For this review, take the finished solid that the model builds, in its own axes (mm). A direction names the side the tool comes from. Round coordinates to 2 decimals unless told otherwise and drop trailing zeros. Loops run counter-clockwise (first coordinate to the right, second up) from the corner with the lowest first, then second, coordinate; pieces in that order, holes last. Notation, with made-up numbers: M -21.5,65.5 L -7.5,65.5 A27 ccw -7.5,94.5 Z; hole C 12.5,73 d6. An arc over 180 degrees is marked long. One line per question, with ' | ' between items. Start each with the question number.
1) For pin 1 Ø10 at (x, y) = (-11.5, -30) entering from +Z; pin 2 Ø1 at (x, z) = (-10, 48) entering from +Y; pin 3 Ø13.5 at (x, y) = (-6, 9.5) entering from +Z; pin 4 Ø10 at (x, y) = (-10.5, 26.5) entering from -Z, all flat-tipped, find the tip position at first contact; note any pin that passes through.
2) We need section D-D (x = -18). Give the boundary of the cut face in (y, z), and give its area (3 significant figures).
3) For probe 1 along Z at (x, y) = (-6.5, -12.5); probe 2 along Y at (x, z) = (5, 24); probe 3 along Y at (x, z) = (-5.5, 5.5), list the stretches that pass through material, from the lowest coordinate up. Write a range as from..to.
4) We need section C-C (x = 6.5). Give the boundary of the cut face in (y, z), and give its area (3 significant figures).
5) We need section A-A (z = 52). Give the boundary of the cut face in (x, y), and give its area (3 significant figures).
6) Mouldability with a two-part tool opening along Z and no side actions: class faces 3 (the face through (10, 0, 10)), 4 (the face through (0, -37.5, 43)), 5 (the face through (0, -9, 0)), 6 (the face through (-12.558, -41.198, 27.976)) as pulls with the +Z half, pulls with the -Z half, needs draft (parallel to the pull), parting line crosses it, or undercut.
7) We need section B-B (y = 7.5). Give the boundary of the cut face in (x, z), and give its area (3 significant figures).
8) For faces 1 (the face through (0, -41, 70)), 2 (the face through (12.558, -41.198, 27.976)), list the 3-axis set-ups (+Z, -Z, +X, -X, +Y, -Y) from which the entire face can be reached by the end or side of a thin tool; tool diameter is ignored.
```python
from build123d import *

# Parameters (mm, degrees)
SKETCH1_W           = 45
SKETCH1_H           = 90
BOSS_EXTRUDE1_DEPTH = 10
SKETCH2_R           = 16
CUT_EXTRUDE1_DEPTH  = 28
FILLET1_R           = 10
SKETCH3_W           = 45
SKETCH3_H           = 7.5
BOSS_EXTRUDE2_DEPTH = 60
FILLET2_R           = 7.5
CUT_EXTRUDE2_DEPTH  = 10


with BuildPart() as part:
    # Sketch1 → Boss-Extrude1 (new body)
    with BuildSketch(Plane.XY):
        Rectangle(SKETCH1_W, SKETCH1_H)
    extrude(amount=BOSS_EXTRUDE1_DEPTH)

    # Sketch2 → Cut-Extrude1 (cut)
    with BuildSketch(Plane.XY):
        with Locations((0.129474069, 13.005480981)):
            Circle(SKETCH2_R)
    extrude(amount=CUT_EXTRUDE1_DEPTH, mode=Mode.SUBTRACT)

    # Fillet1
    fillet1_edges = [part.edges().sort_by_distance(p)[0] for p in [
        (-22.5, 45, 5),
        (22.5, 45, 5),
    ]]
    fillet(fillet1_edges, radius=FILLET1_R)

    # Sketch3 → Boss-Extrude2 (add)
    with BuildSketch(Plane.XY.offset(10)):
        with Locations((0, -41.25)):
            Rectangle(SKETCH3_W, SKETCH3_H)
    extrude(amount=BOSS_EXTRUDE2_DEPTH)

    # Fillet2
    fillet2_edges = [part.edges().sort_by_distance(p)[0] for p in [
        (0, -37.5, 10),
    ]]
    fillet(fillet2_edges, radius=FILLET2_R)

    # Sketch4 → Cut-Extrude2 (cut)
    with BuildSketch(Plane(origin=(0, -37.5, 0), x_dir=(1, 0, 0), z_dir=(0, 1, 0))):
        with BuildLine():
            Line((-9.85, -30.625), (-9.85, -60.625))
            ThreePointArc((-9.85, -60.625), (-12.5, -63.275), (-15.15, -60.625))
            Line((-15.15, -60.625), (-15.15, -30.625))
            ThreePointArc((-15.15, -30.625), (-12.5, -27.975), (-9.85, -30.625))
        make_face()
        with BuildLine():
            Line((9.85, -30.625), (9.85, -60.625))
            ThreePointArc((9.85, -60.625), (12.5, -63.275), (15.15, -60.625))
            Line((15.15, -60.625), (15.15, -30.625))
            ThreePointArc((15.15, -30.625), (12.5, -27.975), (9.85, -30.625))
        make_face()
    extrude(amount=-CUT_EXTRUDE2_DEPTH, mode=Mode.SUBTRACT)


solid = part.part
```
Answers below:
1) pin 1: z = 11.91 | pin 2: y = -37.5 | pin 3: through | pin 4: z = 0
2) outline: M -45,0 L 43.35,0 L 43.35,10 L -30,10 A7.5 cw -37.5,17.5 L -37.5,70 L -45,70 Z | area: 1,350 mm^2
3) probe 1: 0..10 | probe 2: -45..-37.5 | probe 3: -45..-1.97, 27.98..45
4) outline: M -45,0 L -1.67,0 L -1.67,10 L -30,10 A7.5 cw -37.5,17.5 L -37.5,70 L -45,70 Z; M 27.68,0 L 45,0 L 45,10 L 27.68,10 Z | area: 1,070 mm^2
5) outline: M -22.5,-45 L -15.15,-45 L -15.15,-37.5 L -22.5,-37.5 Z; M -9.85,-45 L 9.85,-45 L 9.85,-37.5 L -9.85,-37.5 Z; M 15.15,-45 L 22.5,-45 L 22.5,-37.5 L 15.15,-37.5 Z | area: 258 mm^2
6) face 3: pulls with the +Z half | face 4: needs draft | face 5: pulls with the -Z half | face 6: undercut
7) outline: M -22.5,0 L -14.89,0 L -14.89,10 L -22.5,10 Z; M 15.15,0 L 22.5,0 L 22.5,10 L 15.15,10 Z | area: 150 mm^2
8) face 1: +Z, +X, -X, +Y, -Y | face 2: +Y, -Y
